Input: dimensioned drawing with shaded views. Units: mm. Origin: part minimum x, y, z. A direction names the side the tool comes from. Round coordinates to 2 decimals unless told otherwise and drop trailing zeros. Order: outer loops, then holes, each group sorted by start corner. A loop starts at its lowest first (then second) coordinate and runs counter-clockwise, first axis right, second up.
Item 1: Cut plane C-C on x = 86. Output: boundary loops of the cut face in (y, z).
Item 2: Cut plane A-A on y = 4. Output: boundary loops of the cut face in (x, z), then the cut area to 3 significant figures.
Item 3: Reachability of the marked faces 1 and 2 from +Z, -Z, +X, -X, +Y, -Y: full face, straight path, thin tool, end or side. Return the list, or none.
Item 4: Line query: L1, parallel to X at y = 7.75, z = 6.75; L2, parallel to Y at x = 30, z = 3.75; L3, parallel to Z at x = 87.5, y = 5. Output: solid intervals per line, ascending.
Item 5: First-contact query: pin 1 (2 mm diameter, centred on x = 43.5, z = 4.5, fed in from +Y); pin 2 (2 mm diameter, centred on x = 87.5, y = 4.5, fed in from -Z). Flat tips, straight axial feed; report the tip coordinate or a pass-through.
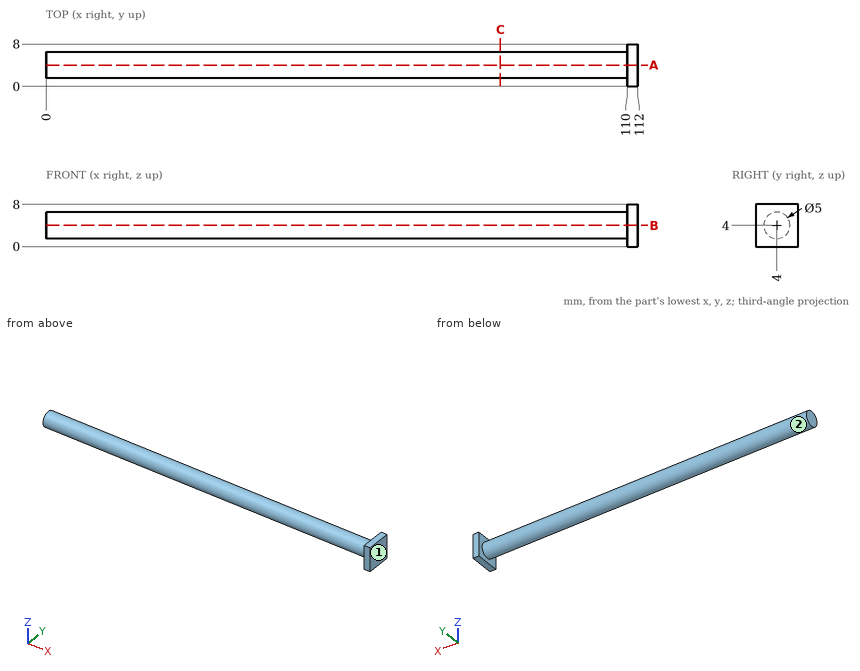
From the geometry:
1. outline: circle Ø5 at (4, 4)
2. outline: (0, 1.5) - (110, 1.5) - (110, 0) - (112, 0) - (112, 8) - (110, 8) - (110, 6.5) - (0, 6.5) - close
2. area: 566 mm2
3. face 1: +Z, -Z, +X, +Y, -Y
3. face 2: -X
4. L1: x = 110 to 112
4. L2: y = 1.51 to 6.49
4. L3: z = 1.71 to 6.29
5. pin 1: stops at y = 6.5
5. pin 2: stops at z = 1.5
